Autodesk Fusion 360 part; units mm, degrees
sketch "Sketch1" plane through (0, 0, 0) normal (0, 1, 0) x (1, 0, 0)
  line L0 (-33, 47) -> (33, 47)
  line L1 (33, 47) -> (33, 41)
  line L2 (33, 41) -> (50, 41)
  line L3 (50, 41) -> (50, 0)
  line L4 (-50, 0) -> (-50, 41)
  line L5 (-50, 41) -> (-33, 41)
  line L6 (-33, 41) -> (-33, 47)
  arc A0 (20, 0) -> (-20, 0) centre (0, 0) ccw
  line L7 (50, 0) -> (20, 0)
  line L8 (-20, 0) -> (-50, 0)
  line L9 (50, 35) -> (35, 35)
  line L10 (35, 35) -> (35, 20)
  line L11 (35, 20) -> (50, 20)
  line L12 (50, 20) -> (50, 35)
  line L13 (-50, 35) -> (-35, 35)
  line L14 (-35, 35) -> (-35, 20)
  line L15 (-35, 20) -> (-50, 20)
  line L16 (-50, 20) -> (-50, 35)
  line L17 (-50, 35) -> (50, 35)
  dimension "d1" = 100
  dimension "d2" = 47
  dimension "d3" = 17
  dimension "d4" = 6
  dimension "d5" = 40
  dimension "d6" = 50
  dimension "d7" = 15
  dimension "d8" = 15
  dimension "d9" = 6
extrude "Extrude1" add sketch "Sketch1" along normal blind 80 contours L0 L1 L2 L3 L4 L5 L6 L9 L13 L17
extrude "Extrude2" add sketch "Sketch1" along normal blind 80 contours L4 L13 L14 L15 L16 L17 | L3 L9 L10 L11 L12 L17
extrude "Extrude3" add sketch "Sketch1" along normal blind 20 contours L3 L4 A0 L7 L8 L10 L11 L14 L15 L17
chamfer "Chamfer1" distance 12 distance2 4 1 edges at (50, 10, 0) measured on face at (40, 6.6667, 0)
chamfer "Chamfer2" distance 4 distance2 12 1 edges at (-50, 10, 0) measured on face at (-50, 33.3333, -34)
chamfer "Chamfer3" distance 15 distance2 60 2 edges at (42.5, 80, -20) (-42.5, 80, -20) measured on face at (45, 80, -32) measured on face at (45, 80, -32)
sketch "Sketch2" plane through (0, 0, -35) normal (0, 0, 1) x (-1, 0, 0)
  line L0 (35, -20) -> (-35, -20)
  line L1 (-35, -20) -> (-35, -80)
  line L2 (-35, -80) -> (35, -80)
  line L3 (35, -80) -> (35, -20)
  line L4 (20, -45) -> (-20, -45)
  arc A0 (-20, -45) -> (-20, -55) centre (-20, -50) ccw
  line L5 (-20, -55) -> (20, -55)
  arc A1 (20, -55) -> (20, -45) centre (20, -50) ccw
  line L6 (25, -50) -> (-25, -50) construction
  line L7 (50, -80) -> (50, -20)
  dimension "d22" = 5
  dimension "d23" = 30
  dimension "d24" = 40
  dimension "d25" = 30
extrude "Extrude4" cut sketch "Sketch2" along normal through all contours L4 A0 L5 A1
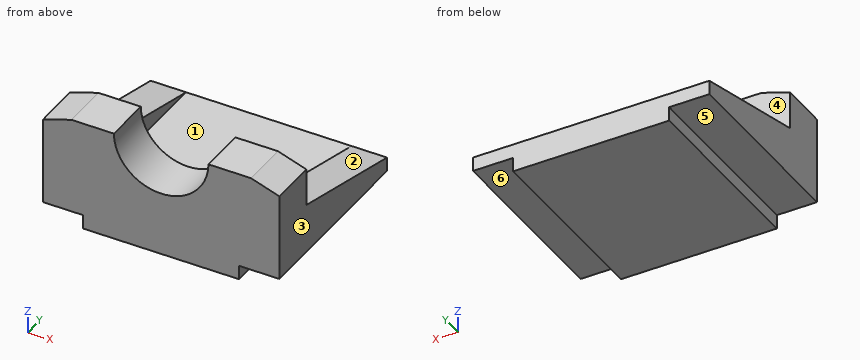
Here's how the part is built. I have some questions about the finished solid (model axes, mm). Face numbers are marked on the shaded views. A direction names the side the tool comes from. Coordinates: 2 decimals unless noted, no trailing zeros. Loops run counter-clockwise (first coordinate to the right, second up) from the corner with the lowest first, then second, coordinate; pieces in that order, holes last.
1. I need wall thicknesses on L1, parallel to X at y = 32, z = -31.5; L2, parallel to Y at x = -39.5, z = -9.5; L3, parallel to Z at x = -22, y = 30.5. Which ranges of each line are inside material? Lowest first, please.
2. If we mould it in two halves opening along X, with no side actions, what happens to the marked faces 1, 2 and 3? For each: pulls with the +X half, pulls with the -X half, needs draft (parallel to the pull), parting line crosses it, or undercut.
3. For the marked faces 4, 5 and 6, which set-ups out of +Z, -Z, +X, -X, +Y, -Y let a thin tool reach every point of the face, with its end or its side?
4. Imagine slicing it at A-A, the plane z = -6.5. Please give me the cut outline in (x, y).
5. Imagine slicing it at B-B, the plane y = 18. Please give me the cut outline in (x, z), and give its area (3 significant figures).
6. Imagine slicing it at D-D, the plane x = 0. Please give me the cut outline in (y, z).
7. Imagine slicing it at C-C, the plane z = -28.5. Please give me the cut outline in (x, y).
8. For P1, Ø5, axis at x = 20.5, z = -34, coming from the -Y side; P2, Ø3, axis at x = -11, y = 57, coming from the +Z side; P3, Ø1.8, axis at y = 50, z = -45, coming from the +X side; P4, Ø1.8, axis at y = 36, z = -45, coming from the -X side, each with a flat end and sliding along its axis, tell me the tip position at first contact or that it passes through.
Taken from the geometry:
1. L1: x = -50 to -35, 35 to 50
1. L2: y = 0 to 20
1. L3: z = -47 to -35
2. face 1: undercut
2. face 2: needs draft
2. face 3: pulls with the +X half
3. face 4: +Z, +Y
3. face 5: -Z, -X, +Y, -Y
3. face 6: -Z, +X, +Y, -Y
4. outline: (-50, 0) - (-18.91, 0) - (-18.91, 20) - (-50, 20) - close; (18.91, 0) - (50, 0) - (50, 20) - (18.91, 20) - close
5. outline: (-50, -41) - (-33, -41) - (-33, -47) - (33, -47) - (33, -41) - (50, -41) - (50, -4) - (38, 0) - (20, 0) arc R20 cw to (-20, 0) - (-38, 0) - (-50, -4) - close
5. area: 3,820 mm2
6. outline: (0, -47) - (80, -47) - (80, -35) - (20, -35) - (20, -20) - (0, -20) - close
7. outline: (-50, 0) - (50, 0) - (50, 54.01) - (35, 54.01) - (35, 20) - (-35, 20) - (-35, 54.01) - (-50, 54.01) - close
8. P1: stops at y = 0
8. P2: stops at z = -35
8. P3: stops at x = 33
8. P4: stops at x = -33
